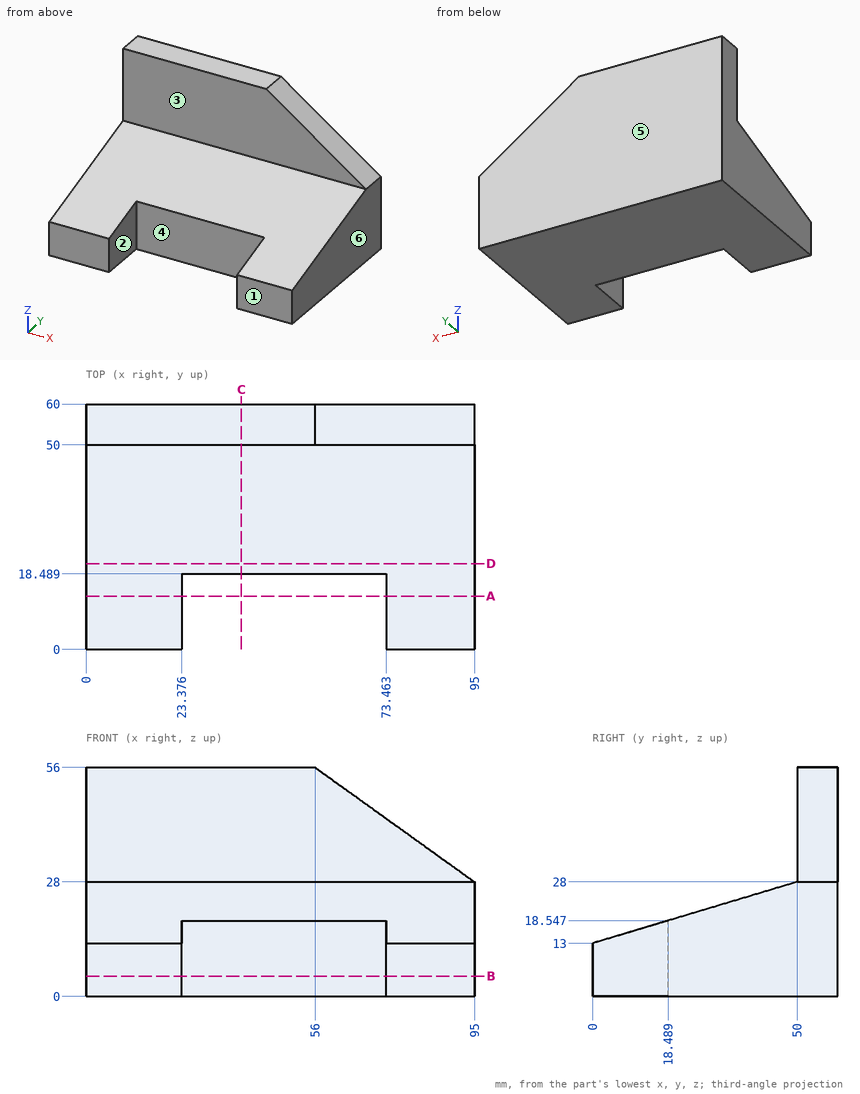
Could you check a few things on this drawing? It's one solid part, dimensions in mm from its lowest x, y, z. A direction names the side the tool comes from. Coordinates: 2 decimals unless noted, no trailing zeros. Write each loop counter-clockwise with the first axis right and the second up, starting at its lowest first coordinate (ties: lowest second). Pieces come first, ordered by that corner, then holes. Notation, with made-up numbers: (-37.75, 31) - (13.25, 31) arc R15 ccw to (13.25, 44) - close; hole circle Ø3 at (61.25, -4.75). An arc over 180 degrees is marked (long way). Return JSON: item names as keys, results as strings. Group by question number.
Item 1: Please list where these lines run through material, in increasing order: probe 1 along X at (y, z) = (17.5, 7); probe 2 along Y at (x, z) = (53, 36); probe 3 along Y at (x, z) = (54.5, 3).
Item 2: If we section it at D-D (y = 21): Write out the boundary of the cut face in (x, z), then the cut area to 3 significant figures.
Item 3: Which directions (+Z, -Z, +X, -X, +Y, -Y) give clear straight access to the entire face, cutting with the end or side of a thin tool? Please do the marked faces 1, 2 and 3.
Item 4: If we section it at B-B (z = 5): Write out the boundary of the cut face in (x, y), then the cut area to 3 significant figures.
Item 5: I'm going to push flat-ended pins straight in: pin 1 Ø22.5 at (x, z) = (57.5, 45) entering from -Y; pin 2 Ø5.5 at (x, z) = (54, 12.5) entering from -Y. Where does each tip first touch, or does it pass through?
Item 6: If we section it at C-C (x = 38): Write out the boundary of the cut face in (y, z).
Item 7: We'd pull the mould along X, two halves only. Please class the marked faces 4, 5 and 6: pulls with the +X half, pulls with the -X half, needs draft (parallel to the pull), parting line crosses it, or undercut.
Item 8: If we section it at A-A (y = 13): Write out the boundary of the cut face in (x, z).
Return value:
{
 "1": {"probe 1": "x = 0 to 23.38, 73.46 to 95", "probe 2": "y = 50 to 60", "probe 3": "y = 18.49 to 60"},
 "2": {"outline": "(0, 0) - (95, 0) - (95, 19.3) - (0, 19.3) - close", "area": "1,830 mm^2"},
 "3": {"face 1": "+Z, -Z, +X, -X, -Y", "face 2": "+Z, -Z, -Y", "face 3": "+Z, +X, -X, -Y"},
 "4": {"outline": "(0, 0) - (23.38, 0) - (23.38, 18.49) - (73.46, 18.49) - (73.46, 0) - (95, 0) - (95, 60) - (0, 60) - close", "area": "4,770 mm^2"},
 "5": {"pin 1": "stops at y = 50", "pin 2": "stops at y = 18.49"},
 "6": {"outline": "(18.49, 0) - (60, 0) - (60, 56) - (50, 56) - (50, 28) - (18.49, 18.55) - close"},
 "7": {"face 4": "undercut", "face 5": "needs draft", "face 6": "pulls with the +X half"},
 "8": {"outline": "(0, 0) - (23.38, 0) - (23.38, 16.9) - (0, 16.9) - close; (73.46, 0) - (95, 0) - (95, 16.9) - (73.46, 16.9) - close"}
}
